Verification items for the finished model (mm, model axes). A direction names the side the tool comes from. Coordinates: 2 decimals unless noted, no trailing zeros. Loops run counter-clockwise (first coordinate to the right, second up) from the corner with the lowest first, then second, coordinate; pieces in that order, holes last.
Q1. Access from +Z, -Z, +X, -X, +Y, -Y to the whole of each face (thin tool, end or side, straight path). Record for faces 1 (the face through (50, 2, -66)), 2 (the face through (85, 3, -43)), 3 (the face through (75, 2, -67)), 4 (the face through (-23, 2, 47)).
Q2. Sectioned sample at A-A (z = -1). Enter the section's corners in (x, y).
Q3. Mould release check, pull along Z, two halves, no side actions. Record for faces 5 (the face through (82, 2, -63)), 6 (the face through (6, 0, 2)), 7 (the face through (82, 3, -58)), 8 (the face through (-42.72, 2.535, 5.274)): +Z half, -Z half, draft (parallel to the pull), parting line (faces both ways), or undercut.
Q4. Go/stop test with flat-tipped pins: P1, Ø2.5, axis at y = 3, z = -65, coming from the +X side; P2, Ø2.5, axis at x = 83, y = 2.5, coming from the +Z side; P3, Ø2.5, axis at x = 8, y = 1.5, coming from the +Z side. Record where each tip stops, or that it passes through.
Q5. Sectioned sample at C-C (z = -15). Enter the section's corners in (x, y).
Q6. Sectioned sample at D-D (x = 54.1). Enter the section's corners in (y, z), then the cut area to 3 significant figures.
Q7. Material ranges on probe 1 along X at (y, z) = (1.1, -25); probe 2 along X at (y, z) = (3.15, -19); probe 3 along Z at (x, y) = (0, 0.95), recorded low to high.
Q8. Sectioned sample at B-B (y = 4.2). Enter the section's corners in (x, z), then the cut area to 3 significant figures.
```python
from build123d import *

# Parameters (mm, degrees)
BOSS_EXTRUDE1_DEPTH = 5
CUT_EXTRUDE1_DEPTH  = 6
CUT_EXTRUDE2_DEPTH  = 6
SKETCH6_W           = 5
SKETCH6_H           = 30
CUT_EXTRUDE4_DEPTH  = 6
CUT_EXTRUDE5_DEPTH  = 6


with BuildPart() as part:
    # Sketch1 → Boss-Extrude1 (new body)
    with BuildSketch(Plane(origin=(0, 0, 0), x_dir=(1, 0, 0), z_dir=(0, 1, 0))):
        with BuildLine():
            Line((-90, -43), (-90, 63))
            Line((-90, 63), (50, 63))
            Line((50, 63), (50, 70))
            Line((50, 70), (75, 70))
            Line((75, 70), (75, 63))
            Line((75, 63), (90, 63))
            Line((90, 63), (90, 13.132821453))
            ThreePointArc((90, 13.132821453), (26.02369403, 21.167044845), (19.690698932, -43))
            Line((19.690698932, -43), (2, -43))
            Line((2, -43), (2, -50))
            Line((2, -50), (-23, -50))
            Line((-23, -50), (-23, -43))
            Line((-23, -43), (-90, -43))
        make_face()
    extrude(amount=BOSS_EXTRUDE1_DEPTH)

    # Sketch2 → Cut-Extrude1 (cut, through all)
    with BuildSketch(Plane(origin=(0, 5, 0), x_dir=(1, 0, 0), z_dir=(0, 1, 0))):
        Polygon((-90, -43), (20.646102312, 63), (-90, 63), align=None)
    extrude(amount=-CUT_EXTRUDE1_DEPTH, mode=Mode.SUBTRACT)

    # Sketch4 → Cut-Extrude2 (cut, through all)
    with BuildSketch(Plane(origin=(0, 5, 0), x_dir=(1, 0, 0), z_dir=(0, 1, 0))):
        Polygon((-1.099353578, 38.01312996), (-44.425657525, -3.493874103), (-40.966740519, -7.104399432), (2.359563427, 34.402604632), (3.081668493, 35.094388033), (-0.377248513, 38.704913361), align=None)
    extrude(amount=-CUT_EXTRUDE2_DEPTH, mode=Mode.SUBTRACT)

    # Sketch6 → Cut-Extrude4 (cut, through all)
    with BuildSketch(Plane(origin=(0, 5, 0), x_dir=(1, 0, 0), z_dir=(0, 1, 0))):
        with Locations((82.5, 43)):
            Rectangle(SKETCH6_W, SKETCH6_H)
    extrude(amount=-CUT_EXTRUDE4_DEPTH, mode=Mode.SUBTRACT)

    # Sketch8 → Cut-Extrude5 (cut, through all)
    with BuildSketch(Plane(origin=(0, 5, 0), x_dir=(1, 0, 0), z_dir=(0, 1, 0))):
        Polygon((-81.041343938, -43), (-81.041343938, -34.417523775), (-90, -43), align=None)
    extrude(amount=-CUT_EXTRUDE5_DEPTH, mode=Mode.SUBTRACT)


solid = part.part
```
Geometry check:
1. face 1: -Z, -X, +Y, -Y
1. face 2: +Y, -Y
1. face 3: -Z, +X, +Y, -Y
1. face 4: +Z, -X, +Y, -Y
2. outline: (-44.07, 0) - (-39.73, 0) - (-39.73, 5) - (-44.07, 5) - close; (-32.51, 0) - (11.67, 0) - (11.67, 5) - (-32.51, 5) - close
3. face 5: -Z half
3. face 6: draft
3. face 7: undercut
3. face 8: undercut
4. P1: stops at x = 75
4. P2: stops at z = -19.41
4. P3: stops at z = 43
5. outline: (-29.46, 0) - (-25.12, 0) - (-25.12, 5) - (-29.46, 5) - close; (-17.89, 0) - (19.69, 0) - (19.69, 5) - (-17.89, 5) - close; (88.51, 0) - (90, 0) - (90, 5) - (88.51, 5) - close
6. outline: (0, -70) - (5, -70) - (5, -31) - (0, -31) - close
6. area: 195 mm2
7. probe 1: x = -19.02 to -14.68, -7.46 to 31.65, 76.55 to 90
7. probe 2: x = -25.28 to -20.95, -13.72 to 23.51, 84.69 to 90
7. probe 3: z = -43.22 to -38.31, -32.14 to 50
8. outline: (-81.04, 34.42) - (20.65, -63) - (50, -63) - (50, -70) - (75, -70) - (75, -63) - (90, -63) - (90, -13.13) arc R45 cw (long way) to (19.69, 43) - (2, 43) - (2, 50) - (-23, 50) - (-23, 43) - (-81.04, 43) - close; hole (-44.43, 3.49) - (-0.38, -38.7) - (3.08, -35.09) - (-40.97, 7.1) - close; hole (80, -58) - (85, -58) - (85, -28) - (80, -28) - close
8. area: 7,810 mm2
